Could you check a few things on this drawing? It's one solid part, dimensions in mm from its lowest x, y, z. A direction names the side the tool comes from. Give positions to 0.01 mm unless a question says otherwise; leave off trailing zeros. Order: outer loops, then holes, each group sorted by start corner. A loop starts at its lowest first (then second) coordinate and runs counter-clockwise, first axis right, second up. Notation, with made-up numbers: (8, -23) - (27, -23) arc R31 ccw to (27, 14) - close; hole circle Ø11 at (46.5, 59.5). An arc over 180 degrees is marked (long way). Put each result on its own line as item: value.
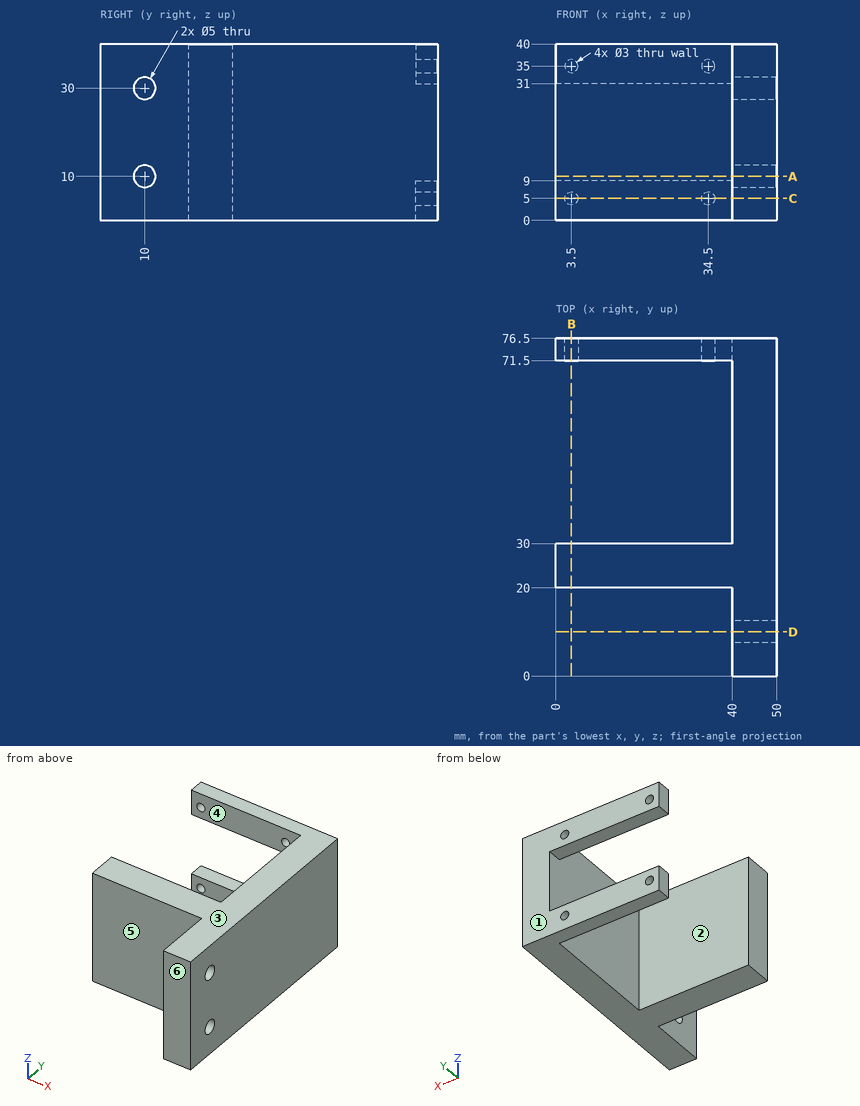
1) I'm going to push flat-ended pins straight in: pin 1 (12 mm diameter, centred on y = 48.5, z = 21.5, fed in from -X); pin 2 (2 mm diameter, centred on x = 30, z = 23, fed in from -Y); pin 3 (2.5 mm diameter, centred on x = 34.5, z = 5, fed in from +Y); pin 4 (3 mm diameter, centred on y = 10, z = 10, fed in from -X). Where does each tip first touch, or does it pass through?
Filled in:
pin 1: stops at x = 40
pin 2: stops at y = 20
pin 3: stops at y = 30
pin 4: passes through
2) If I drill on line 1 (Z direction, x = 3.5, y = 73.65); line 2 (Z direction, x = 32, y = 72); line 3 (X direction, y = 73, z = 5), over which ranges is the centre line in solid material (lowest first)? Write a range as [from, to].
Filled in:
line 1: z = [0, 3.5], [6.5, 9], [31, 33.5], [36.5, 40]
line 2: z = [0, 9], [31, 40]
line 3: x = [0, 2], [5, 33], [36, 50]
3) Suppose I cut it at C-C, the plane z = 5. List the corners of the cut face in (x, y) for me, and give its area (4 significant figures).
Filled in:
outline: (0, 20) - (40, 20) - (40, 0) - (50, 0) - (50, 76.5) - (36, 76.5) - (36, 71.5) - (40, 71.5) - (40, 30) - (0, 30) - close; (0, 71.5) - (2, 71.5) - (2, 76.5) - (0, 76.5) - close; (5, 71.5) - (33, 71.5) - (33, 76.5) - (5, 76.5) - close
area: 1,335 mm^2
4) We'd pull the mould along Y, two halves only. Please class the marked faces 1, 2 and 3: pulls with the +Y half, pulls with the -Y half, needs draft (parallel to the pull), parting line crosses it, or undercut.
Filled in:
face 1: pulls with the +Y half
face 2: undercut
face 3: needs draft
5) Suppose I cut it at D-D, the plane y = 10. List the corners of the cut face in (x, z) for me, and give its area (3 significant figures).
Filled in:
outline: (40, 0) - (50, 0) - (50, 7.5) - (40, 7.5) - close; (40, 12.5) - (50, 12.5) - (50, 27.5) - (40, 27.5) - close; (40, 32.5) - (50, 32.5) - (50, 40) - (40, 40) - close
area: 300 mm^2
6) Suppose I cut it at B-B, the plane x = 3.5. List the corners of the cut face in (y, z) for me.
Filled in:
outline: (20, 0) - (30, 0) - (30, 40) - (20, 40) - close; (71.5, 0) - (76.5, 0) - (76.5, 3.5) - (71.5, 3.5) - close; (71.5, 6.5) - (76.5, 6.5) - (76.5, 9) - (71.5, 9) - close; (71.5, 31) - (76.5, 31) - (76.5, 33.5) - (71.5, 33.5) - close; (71.5, 36.5) - (76.5, 36.5) - (76.5, 40) - (71.5, 40) - close
7) Which directions (+Z, -Z, +X, -X, +Y, -Y) give clear straight access to the entire face, cutting with the end or side of a thin tool? Please do the marked faces 4, 5 and 6.
Filled in:
face 4: +Z, -Z, -X
face 5: +Z, -Z, -X, -Y
face 6: +Z, -Z, +X, -X, -Y
8) Suppose I cut it at A-A, the plane z = 10. List the corners of the cut face in (x, y) for me.
Filled in:
outline: (0, 20) - (40, 20) - (40, 12.5) - (50, 12.5) - (50, 76.5) - (40, 76.5) - (40, 30) - (0, 30) - close; (40, 0) - (50, 0) - (50, 7.5) - (40, 7.5) - close
